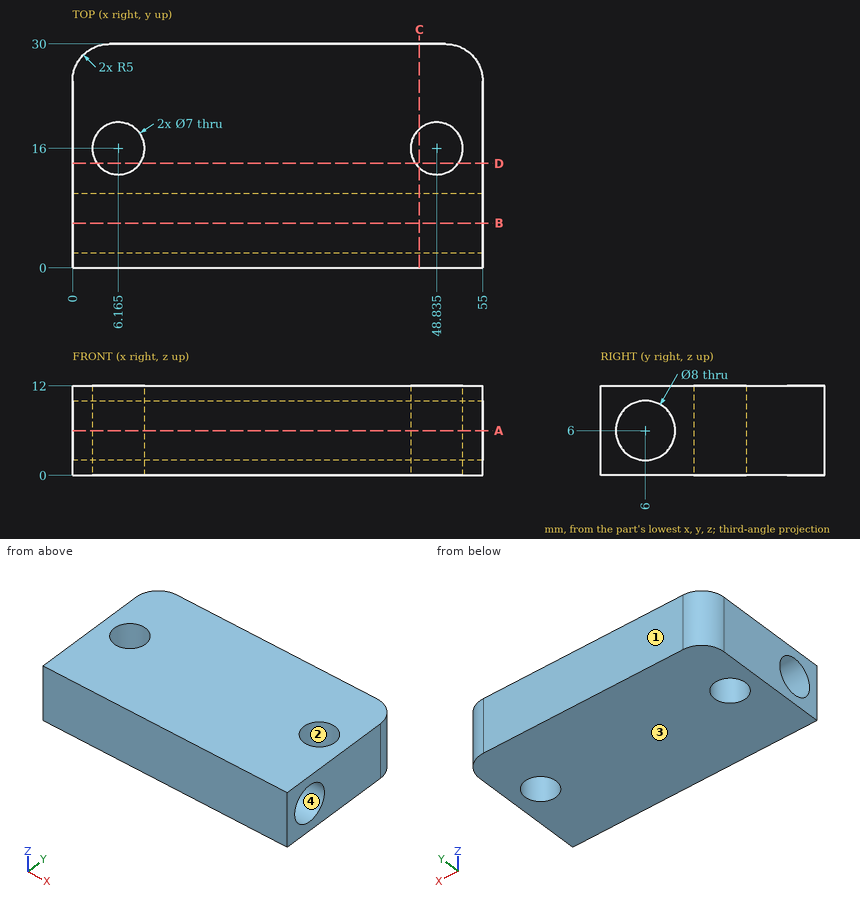
Geometry: see drawing. Coordinates: mm, zero at the bounding-box minimum. Coordinates: 2 decimals unless noted, no trailing zeros. Loops run counter-clockwise (first coordinate to the right, second up) from the corner with the lowest first, then second, coordinate; pieces in that order, holes last.
(1) First-contact query: pin 1 Ø1.5 at (y, z) = (8.5, 6) entering from -X. Flat tip, straight axial feed; report the tip coordinate or a pass-through.
(2) Material intervals for probe 1 along Y at (x, z) = (32, 6); probe 2 along Y at (x, z) = (9, 3); probe 3 along X at (y, z) = (19, 8.75), sorted ascending.
(3) Section B-B on y = 6. Return the cut outline in (x, z), then the cut area to 3 significant figures.
(4) Section C-C on x = 46.5. Return the cut outline in (y, z).
(5) Pull-direction query (Y, two-part tool) for the marked faces 1, 2, 3 and 4; classes: released by +Y, released by -Y, zero draft, split by the parting line, or undercut.
(6) Section A-A on z = 6. Return the cut outline in (x, y) (3 decimals).
(7) Section D-D on y = 14. Return the cut outline in (x, z), then the cut area to 3 significant figures.
Data:
1. pin 1: passes through
2. probe 1: y = 0 to 2, 10 to 30
2. probe 2: y = 0 to 3.35, 8.65 to 13.95, 18.05 to 30
2. probe 3: x = 0 to 4.36, 7.97 to 47.03, 50.64 to 55
3. outline: (0, 0) - (55, 0) - (55, 2) - (0, 2) - close; (0, 10) - (55, 10) - (55, 12) - (0, 12) - close
3. area: 220 mm2
4. outline: (0, 0) - (13.39, 0) - (13.39, 12) - (0, 12) - close; (18.61, 0) - (30, 0) - (30, 12) - (18.61, 12) - close; hole circle Ø8 at (6, 6)
5. face 1: released by +Y
5. face 2: undercut
5. face 3: zero draft
5. face 4: undercut
6. outline: (0, 0) - (55, 0) - (55, 2) - (0, 2) - close; (0, 10) - (55, 10) - (55, 25) arc R5 ccw to (50, 30) - (5, 30) arc R5 ccw to (0, 25) - close; hole circle Ø7 at (6.165, 16); hole circle Ø7 at (48.835, 16)
7. outline: (0, 0) - (3.29, 0) - (3.29, 12) - (0, 12) - close; (9.04, 0) - (45.96, 0) - (45.96, 12) - (9.04, 12) - close; (51.71, 0) - (55, 0) - (55, 12) - (51.71, 12) - close
7. area: 522 mm2
